from build123d import *

# Parameters (mm, degrees)
F0_W     = 42.3
F0_H     = 42.3
F1_DEPTH = 34
F2_R     = 11
F2_R_2   = 3.5
F3_DEPTH = 2
F4_R     = 2.5
F5_DEPTH = 24
F6_SIZE  = 0.5
F7_R     = 1.5
F8_DEPTH = 5
F9_SIZE  = 6


with BuildPart() as f1:
    # F0 (on Top) → F1 (new body)
    with BuildSketch(Plane.XY):
        Rectangle(F0_W, F0_H)
    extrude(amount=F1_DEPTH)

    # F2 (on face) → F3 (join)
    with BuildSketch(Plane.XY.offset(34)):
        Circle(F2_R)
        Circle(F2_R_2, mode=Mode.SUBTRACT)
    extrude(amount=F3_DEPTH)

    # F4 (on face) → F5 (join)
    with BuildSketch(Plane.XY.offset(34)):
        Circle(F4_R)
    extrude(amount=F5_DEPTH)

    # F6
    f6_edges = [f1.edges().sort_by_distance(p)[0] for p in [
        (-2.5, 0, 58),
    ]]
    chamfer(f6_edges, length=F6_SIZE)

    # F7 (on face) → F8 (cut)
    with BuildSketch(Plane.XY.offset(34)):
        with Locations((-15.5, 15.5)):
            Circle(F7_R)
        with Locations((-15.5, -15.5)):
            Circle(F7_R)
        with Locations((15.5, 15.5)):
            Circle(F7_R)
        with Locations((15.5, -15.5)):
            Circle(F7_R)
    extrude(amount=-F8_DEPTH, mode=Mode.SUBTRACT)

    # F9
    f9_edges = [f1.edges().sort_by_distance(p)[0] for p in [
        (21.15, -21.15, 17),
        (-21.15, -21.15, 17),
        (21.15, 21.15, 17),
        (-21.15, 21.15, 17),
    ]]
    chamfer(f9_edges, length=F9_SIZE)


solid = f1.part
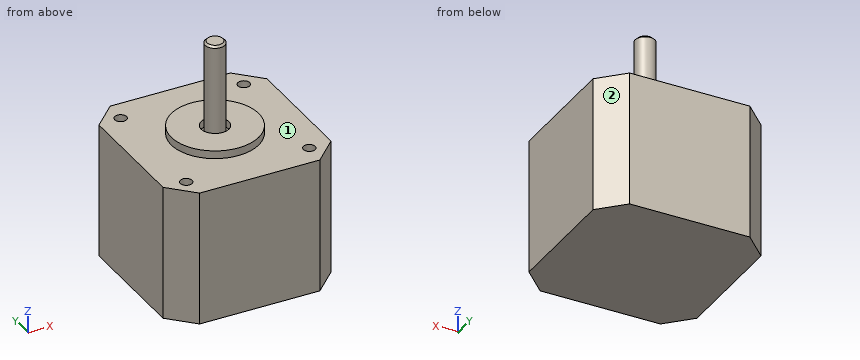
Geometry check sheet. Reference: the model listing, model coordinates, mm. Face numbers are marked on the shaded views. A direction names the side the tool comes from. Round coordinates to 2 decimals unless told otherwise and drop trailing zeros. Order: outer loops, then holes, each group sorted by start corner. A loop starts at its lowest first (then second) coordinate and runs counter-clockwise, first axis right, second up. Notation, with made-up numbers: M 44.25,-5.75 L 70.25,-5.75 A21 ccw 70.25,17.25 Z; hole C -26,11 d4. An arc over 180 degrees is marked long. Answer in a Markdown table with one row per item.
(1) Sectioned sample at A-A, the plane x = 0. Record the cut outline in (y, z), and give its area (3 significant figures).
Responses:
| item | result |
|---|---|
| outline | M -21.15,0 L 21.15,0 L 21.15,34 L 11,34 L 11,36 L 3.5,36 L 3.5,34 L 2.5,34 L 2.5,57.5 L 2,58 L -2,58 L -2.5,57.5 L -2.5,34 L -3.5,34 L -3.5,36 L -11,36 L -11,34 L -21.15,34 Z |
| area | 1,590 mm² |
(2) Scan lines: probe 1 along Y at (x, z) = (15.5, 31); probe 2 along X at (y, z) = (-15, 32); probe 3 along Z at (x, y) = (-18.5, -5). Record each from-to range of solid material in increasing order. Write a range as from..to.
Responses:
| item | result |
|---|---|
| probe 1 | y = -20.8..-17, -14..14, 17..20.8 |
| probe 2 | x = -21.15..-16.91, -14.09..14.09, 16.91..21.15 |
| probe 3 | z = 0..34 |
(3) Go/stop test with flat-tipped pins: P1, Ø3, axis at x = -13, y = -1.5, coming from the +Z side; P2, Ø2.5, axis at x = -15.5, y = 15.5, coming from the +Z side; P3, Ø5, axis at x = -7, y = 4.5, coming from the +Z side. Record where each tip stops, or that it passes through.
Responses:
| item | result |
|---|---|
| P1 | stops at z = 34 |
| P2 | stops at z = 29 |
| P3 | stops at z = 36 |
(4) Sectioned sample at C-C, the plane y = -12. Record the cut outline in (x, z).
Responses:
| item | result |
|---|---|
| outline | M -21.15,0 L 21.15,0 L 21.15,34 L -21.15,34 Z |
(5) Sectioned sample at D-D, the plane y = 8. Record the cut outline in (x, z).
Responses:
| item | result |
|---|---|
| outline | M -21.15,0 L 21.15,0 L 21.15,34 L 7.55,34 L 7.55,36 L -7.55,36 L -7.55,34 L -21.15,34 Z |
(6) Tool access check on the marked faces 1 and 2. Record the directions out of +Z, -Z, +X, -X, +Y, -Y that give a thin tool (end or side, any length) a straight path to the whole face; none if there is none.
Responses:
| item | result |
|---|---|
| face 1 | +Z |
| face 2 | +Z, -Z, +X, +Y |
(7) Sectioned sample at B-B, the plane z = 20.5. Record the cut outline in (x, y).
Responses:
| item | result |
|---|---|
| outline | M -21.15,-15.15 L -15.15,-21.15 L 15.15,-21.15 L 21.15,-15.15 L 21.15,15.15 L 15.15,21.15 L -15.15,21.15 L -21.15,15.15 Z |
